The listing builds one solid part. Answer for the finished solid, in the listing's coordinates (mm). Face numbers are marked on the shaded views. A direction names the side the tool comes from. Coordinates: 2 decimals unless noted, no trailing zeros. Loops run counter-clockwise (first coordinate to the right, second up) from the corner with the lowest first, then second, coordinate; pieces in that order, holes last. Notation, with made-up numbers: M 78,6 L 110,6 A24 cw 110,19 Z; hole C 50.25,8.5 d10. An arc over 180 degrees is marked long. Answer as a JSON object with one key per item and string values. Group by question number.
1. For the marked faces 4 and 5, determine the directions among +Z, -Z, +X, -X, +Y, -Y from which every point of the face is accessible in a straight line to the end or side of a thin tool.
2. A cutting plane is placed at C-C on y = 8. Give the vertices of the cut face in (x, z) (3 decimals).
3. Determine the mould class of the marked faces 1, 2 and 3 for opening direction Y: released by +Y, released by -Y, zero draft, split by the parting line, or undercut.
4. A cutting plane is placed at B-B on x = -2. Give the vertices of the cut face in (y, z), and give its area (3 significant figures).
5. Given pin 1 (7.5 mm diameter, centred on x = 6.5, z = -25.5, fed in from -Y); pin 2 (6 mm diameter, centred on x = -12, z = 10.5, fed in from +Y); pin 3 (3 mm diameter, centred on x = 1.5, z = -28.5, fed in from +Y); pin 4 (1.5 mm diameter, centred on x = 3.5, z = -23.5, fed in from -Y), each flat-ended and moving along its own axis, determine where each tip first touches the part or whether it passes through.
6. Straight lines are drawn through the part: L1, parallel to Z at x = -13.5, y = -4; L2, parallel to Z at x = -6, y = 4.5; L3, parallel to Y at x = 7.5, z = -29. For each, find the intervals that lie inside material, in ascending order.
7. A cutting plane is placed at A-A on y = -2.5. Give the vertices of the cut face in (x, z) (3 decimals), and give its area (3 significant figures).
8. A cutting plane is placed at D-D on z = 0. Give the vertices of the cut face in (x, y) (3 decimals), and give its area (3 significant figures).
Autodesk Inventor part; units mm, degrees
ref_plane "YZ Plane" through (0, 0, 0) normal (1, 0, 0) x (0, 1, 0)
ref_plane "XZ Plane" through (0, 0, 0) normal (0, 1, 0) x (-1, 0, 0)
ref_plane "XY Plane" through (0, 0, 0) normal (0, 0, 1) x (1, 0, 0)
sketch "Sketch1" plane through (0, 0, 0) normal (1, 0, 0) x (0, 1, 0)
  arc A0 (0, -20.32) -> (0, 20.32) centre (0, 0) ccw
  arc A1 (5.08, -24.8868) -> (5.08, 24.8868) centre (0, 0) ccw
  line L0 (0, 25.6032) -> (0, 20.32)
  line L1 (0, -20.32) -> (0, -25.4)
  line L2 (0, 25.6032) -> (0, 29.9668)
  line L3 (0, 29.9668) -> (-6.096, 29.9668)
  line L4 (-6.096, 29.9668) -> (-6.096, 27.4268)
  line L5 (-6.096, 27.4268) -> (-7.62, 28.9508)
  line L6 (-6.096, 27.4268) -> (-3.9407, 27.4268) construction
  line L7 (5.08, 24.8868) -> (5.08, 33.7768)
  line L8 (5.08, 33.7768) -> (-7.62, 33.7768)
  line L9 (-7.62, 33.7768) -> (-7.62, 28.9508)
  line L10 (10.0375, 0) -> (16.2196, 0) construction
  line L11 (0, -25.4) -> (0, -29.9668)
  line L12 (0, -29.9668) -> (-6.096, -29.9668)
  line L13 (-6.096, -29.9668) -> (-6.096, -27.4268)
  line L14 (-6.096, -27.4268) -> (-7.62, -28.9508)
  line L15 (5.08, -24.8868) -> (5.08, -33.7768)
  line L16 (5.08, -33.7768) -> (-7.62, -33.7768)
  line L17 (-7.62, -33.7768) -> (-7.62, -28.9508)
  dimension "d0" = 40.64
  dimension "d1" = 50.8
  dimension "d3" = 6.096
  dimension "d4" = 2.54
  dimension "d5" = 135
  dimension "d6" = 5.08
  dimension "d7" = 0
  dimension "d8" = 8.89
  dimension "d9" = 12.7
  dimension "d12" = 5.08
extrude "Extrusion1" add sketch "Sketch1" along normal mid plane 31.75
properties part number "PistonClip"
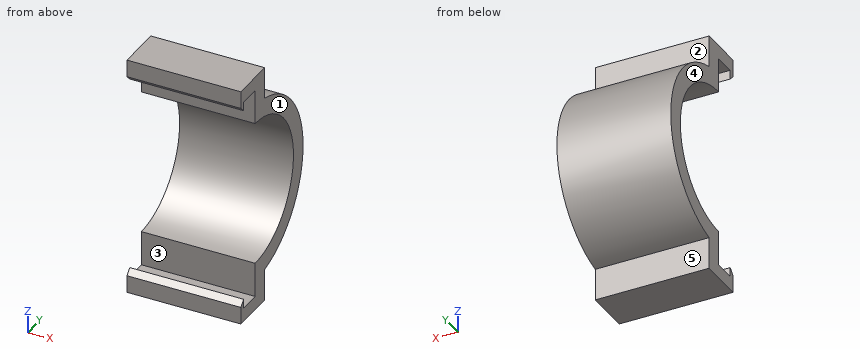
From the geometry:
{
 "1": {"face 4": "+Z, -Z, -X, +Y, -Y", "face 5": "-Z, +X, -X, +Y"},
 "2": {"outline": "M -15.875,-24.107 L 15.875,-24.107 L 15.875,-18.679 L -15.875,-18.679 Z; M -15.875,18.679 L 15.875,18.679 L 15.875,24.107 L -15.875,24.107 Z"},
 "3": {"face 1": "zero draft", "face 2": "released by +Y", "face 3": "undercut"},
 "4": {"outline": "M -7.62,-33.78 L 5.08,-33.78 L 5.08,-24.89 A25.4 ccw 5.08,24.89 L 5.08,33.78 L -7.62,33.78 L -7.62,28.95 L -6.1,27.43 L -6.1,29.97 L 0,29.97 L 0,20.32 A20.32 cw 0,-20.32 L 0,-29.97 L -6.1,-29.97 L -6.1,-27.43 L -7.62,-28.95 Z", "area": "515 mm²"},
 "5": {"pin 1": "stops at y = -7.62", "pin 2": "stops at y = 24.27", "pin 3": "stops at y = 5.08", "pin 4": "stops at y = 0"},
 "6": {"L1": "z = -33.78 to -29.97, 29.97 to 33.78", "L2": "z = -33.78 to -19.82, 19.82 to 33.78", "L3": "y = -7.62 to -6.1, 0 to 5.08"},
 "7": {"outline": "M -15.875,-33.777 L 15.875,-33.777 L 15.875,-29.967 L -15.875,-29.967 Z; M -15.875,29.967 L 15.875,29.967 L 15.875,33.777 L -15.875,33.777 Z", "area": "242 mm²"},
 "8": {"outline": "M -15.875,20.32 L 15.875,20.32 L 15.875,25.4 L -15.875,25.4 Z", "area": "161 mm²"}
}
